CAD build for the part. Positions are in the model's coordinates, mm. A direction names the side the tool comes from. Coordinates: 2 decimals unless noted, no trailing zeros. Loops run counter-clockwise (first coordinate to the right, second up) from the corner with the lowest first, then second, coordinate; pieces in that order, holes last. Notation, with made-up numbers: (23.5, 78) -> (42.5, 78) arc R22 ccw to (42.5, 98) -> close; hole circle Ø9 at (-2.5, -40). An arc over 180 degrees is marked (long way). Return JSON: item names as keys, results as strings. Group by question number.
(1) Flat gauge pin, fed straight in: pin 1 Ø3 at (x, y) = (-14, -8.5) entering from +Z (3 decimals). Where does the tip first touch, or does it go through?
(2) Probe L1, parallel to Z at x = 12.7, y = -15.9 (3 decimals); L2, parallel to Y at x = -1, z = 19. List the from-to ranges inside material, lowest first.
(3) Tool access for faces 1 (the face through (14.288, 0, -12)), 2 (the face through (14.49, 16.02, -53.04)), 3 (the face through (-14.403, -16.024, -52.889)): list every direction of +Z, -Z, +X, -X, +Y, -Y with a clear straight run to the whole face (end or side of a thin tool).
(4) Mould opens along Y. For faces 4 (the face through (0, 19.05, -1)), 5 (the face through (14.49, -16.02, -53.04)), 6 (the face through (-17, 0, 41.275)), 7 (the face through (-14.288, 0, -12)) say: pulls with the +Y half, pulls with the -Y half, needs draft (parallel to the pull), parting line crosses it, or undercut.
(5) Saw through at A-A on z = 7.5. Write the cut outline in (x, y).
```python
from build123d import *

# Parameters (mm, degrees)
SKETCH1_W                       = 38.1
SKETCH1_H                       = 133.35
BOSS_EXTRUDE1_DEPTH             = 19.05
SKETCH2_W                       = 28.575
SKETCH2_H                       = 28.575
CUT_EXTRUDE1_DEPTH              = 134.35
SKETCH3_W                       = 25.4
SKETCH3_H                       = 28.575
CUT_EXTRUDE2_DEPTH              = 39.1
F_10_32_TAPPED_HOLE1_AT_2_COUNT = 2
F_10_32_TAPPED_HOLE1_AT_2_PITCH = 25.4
F_10_32_TAPPED_HOLE1_AT_3_COUNT = 2
F_10_32_TAPPED_HOLE1_AT_3_PITCH = 101.6
F_10_32_TAPPED_HOLE1_AT_4_COUNT = 2
F_10_32_TAPPED_HOLE1_AT_4_PITCH = 104.726882891
F_10_32_TAPPED_HOLE2_D          = 4.0386


with BuildPart() as part:
    # Sketch1 → Boss-Extrude1 (new body, symmetric)
    with BuildSketch(Plane(origin=(0, 0, 0), x_dir=(1, 0, 0), z_dir=(0, 1, 0))):
        Rectangle(SKETCH1_W, SKETCH1_H)
    extrude(amount=BOSS_EXTRUDE1_DEPTH, both=True)

    # Sketch2 → Cut-Extrude1 (cut, through all)
    with BuildSketch(Plane.XY.offset(66.675)):
        Rectangle(SKETCH2_W, SKETCH2_H)
    extrude(amount=-CUT_EXTRUDE1_DEPTH, mode=Mode.SUBTRACT)

    # Sketch3 → Cut-Extrude2 (cut, through all)
    with BuildSketch(Plane(origin=(19.05, 0, 0), x_dir=(0, 0, -1), z_dir=(1, 0, 0))):
        with Locations((-53.975, 0)):
            Rectangle(SKETCH3_W, SKETCH3_H)
    extrude(amount=-CUT_EXTRUDE2_DEPTH, mode=Mode.SUBTRACT)

    # Sketch4 → #10-32 Tapped Hole1 (revolve, cut)
    with BuildSketch(Plane(origin=(-12.7, 19.05, 47.625), x_dir=(0, 0, 1), z_dir=(1, 0, 0))):
        Polygon((0, 0), (0, 12.389317848), (2.0193, 11.176), (2.0193, 0), align=None)
    f_10_32_tapped_hole1 = revolve(axis=Axis((-12.7, 25.4, 47.625), (0, -1, 0)), mode=Mode.SUBTRACT)

    # #10-32 Tapped Hole1 at 2: #10-32 Tapped Hole1 ×2
    with Locations(*[(i * F_10_32_TAPPED_HOLE1_AT_2_PITCH, 0, 0) for i in range(1, F_10_32_TAPPED_HOLE1_AT_2_COUNT)]):
        add(f_10_32_tapped_hole1, mode=Mode.SUBTRACT)

    # #10-32 Tapped Hole1 at 3: #10-32 Tapped Hole1 ×2
    with Locations(*[(0, 0, -i * F_10_32_TAPPED_HOLE1_AT_3_PITCH) for i in range(1, F_10_32_TAPPED_HOLE1_AT_3_COUNT)]):
        add(f_10_32_tapped_hole1, mode=Mode.SUBTRACT)

    # #10-32 Tapped Hole1 at 4: #10-32 Tapped Hole1 ×2
    with Locations(*[Vector(0.242535625, 0, -0.9701425) * (i * F_10_32_TAPPED_HOLE1_AT_4_PITCH) for i in range(1, F_10_32_TAPPED_HOLE1_AT_4_COUNT)]):
        add(f_10_32_tapped_hole1, mode=Mode.SUBTRACT)

    # #10-32 Tapped Hole2 (through all)
    with Locations(Plane(origin=(19.05, 0, 0), x_dir=(0, 0, -1), z_dir=(1, 0, 0))):
        with Locations((0, 0)):
            Hole(F_10_32_TAPPED_HOLE2_D / 2)

    # Mirror1: #10-32 Tapped Hole1 across plane
    add(f_10_32_tapped_hole1.mirror(Plane.ZX), mode=Mode.SUBTRACT)

    # Mirror1 copy 1 sketch → Mirror1 copy 1 (revolve, cut)
    with BuildSketch(Plane(origin=(12.7, -19.05, 47.625), x_dir=(0, 0, 1), z_dir=(1, 0, 0))):
        Polygon((0, 0), (0, -12.389317848), (2.0193, -11.176), (2.0193, 0), align=None)
    revolve(axis=Axis((12.7, -25.4, 47.625), (0, -1, 0)), mode=Mode.SUBTRACT)

    # Mirror1 copy 2 sketch → Mirror1 copy 2 (revolve, cut)
    with BuildSketch(Plane(origin=(-12.7, -19.05, -53.975), x_dir=(0, 0, 1), z_dir=(1, 0, 0))):
        Polygon((0, 0), (0, -12.389317848), (2.0193, -11.176), (2.0193, 0), align=None)
    revolve(axis=Axis((-12.7, -25.4, -53.975), (0, -1, 0)), mode=Mode.SUBTRACT)

    # Mirror1 copy 3 sketch → Mirror1 copy 3 (revolve, cut)
    with BuildSketch(Plane(origin=(12.7, -19.05, -53.975), x_dir=(0, 0, 1), z_dir=(1, 0, 0))):
        Polygon((0, 0), (0, -12.389317848), (2.0193, -11.176), (2.0193, 0), align=None)
    revolve(axis=Axis((12.7, -25.4, -53.975), (0, -1, 0)), mode=Mode.SUBTRACT)


solid = part.part
```
Geometry results:
{
 "1": {"pin 1": "z = 41.275"},
 "2": {"L1": "-66.675 to -55.994, -51.956 to 45.606, 49.644 to 66.675", "L2": "-19.05 to -14.29, 14.29 to 19.05"},
 "3": {"face 1": "+Z, -Z", "face 2": "+Y", "face 3": "-Y"},
 "4": {"face 4": "pulls with the +Y half", "face 5": "needs draft", "face 6": "undercut", "face 7": "undercut"},
 "5": {"outline": "(-19.05, -19.05) -> (19.05, -19.05) -> (19.05, 19.05) -> (-19.05, 19.05) -> close; hole (-14.29, -14.29) -> (14.29, -14.29) -> (14.29, 14.29) -> (-14.29, 14.29) -> close"}
}
